The listing builds one solid part. Answer for the finished solid, in the listing's coordinates (mm). A direction names the side the tool comes from. Round coordinates to 2 decimals unless told otherwise and drop trailing zeros. Write each loop counter-clockwise with the first axis right and the second up, starting at its lowest first coordinate (ties: lowest second). Pieces come first, ordered by that corner, then holes.
(1) Each of these flat-tipped pins is pushed along its axis until it touches: pin 1 Ø1.8 at (x, y) = (-24, 10) entering from -Z; pin 2 Ø6.5 at (x, y) = (0, -23.5) entering from +Z; pin 3 Ø1 at (y, z) = (21, 3) entering from +X; pin 4 Ø1.5 at (x, z) = (14.5, 2) entering from +Y. Where does it stop, or does it pass through?
(2) The mould has two halves that part along Y. Classify faces 3 (the face through (26.327, -10.916, 2.465)), 4 (the face through (-26, 0, 2)), 5 (the face through (19, 9, 5)): +Y half, -Y half, draft (parallel to the pull), parting line (faces both ways), or undercut.
(3) Find the intervals of material crossed by probe 1 along Y at (x, z) = (16, 0.65); probe 2 along X at (y, z) = (15.5, 2.85), in increasing order.
(4) A cutting plane is placed at A-A, the plane x = 0. Give the vertices of the cut face in (y, z), and give its area (3 significant figures).
(5) A cutting plane is placed at D-D, the plane z = 1. Give the number of separate pieces and of enclosed holes in the cut face, and give its area (3 significant figures).
(6) For faces 1 (the face through (21, 0, 2)), 2 (the face through (-10.026, -25.564, 0.986)), determine the directions among +Z, -Z, +X, -X, +Y, -Y from which every point of the face is accessible in a straight line to the end or side of a thin tool.
(7) A cutting plane is placed at C-C, the plane x = 11.5. Give the vertices of the cut face in (y, z), and give its area (3 significant figures).
from build123d import *

# Parameters (mm, degrees)
F0_R     = 28.5
F0_R_2   = 2.5
F0_R_3   = 3
F0_R_4   = 20.5
F1_DEPTH = 5
F2_DEPTH = 2


with BuildPart() as f1:
    # F0 (on Top) → F1 (new body)
    with BuildSketch(Plane.XY):
        Circle(F0_R)
        with Locations((-16.6170093579, -16.6170093579)):
            Circle(F0_R_2, mode=Mode.SUBTRACT)
        with Locations((-9.3757440929, -22.6350485465)):
            Circle(F0_R_3, mode=Mode.SUBTRACT)
        with Locations((-22.6350485465, -9.3757440929)):
            Circle(F0_R_3, mode=Mode.SUBTRACT)
        with Locations((0, -23.5)):
            Circle(F0_R_2, mode=Mode.SUBTRACT)
        with Locations((9.3757440929, -22.6350485465)):
            Circle(F0_R_3, mode=Mode.SUBTRACT)
        with Locations((16.6170093579, -16.6170093579)):
            Circle(F0_R_2, mode=Mode.SUBTRACT)
        with Locations((22.6350485465, -9.3757440929)):
            Circle(F0_R_3, mode=Mode.SUBTRACT)
        with Locations((-23.5, 0)):
            Circle(F0_R_2, mode=Mode.SUBTRACT)
        with Locations((-22.6350485465, 9.3757440929)):
            Circle(F0_R_3, mode=Mode.SUBTRACT)
        with Locations((-16.6170093579, 16.6170093579)):
            Circle(F0_R_2, mode=Mode.SUBTRACT)
        with Locations((-9.3757440929, 22.6350485465)):
            Circle(F0_R_3, mode=Mode.SUBTRACT)
        Circle(F0_R_4, mode=Mode.SUBTRACT)
        with Locations((23.5, 0)):
            Circle(F0_R_2, mode=Mode.SUBTRACT)
        with Locations((22.6350485465, 9.3757440929)):
            Circle(F0_R_3, mode=Mode.SUBTRACT)
        with Locations((0, 23.5)):
            Circle(F0_R_2, mode=Mode.SUBTRACT)
        with Locations((9.3757440929, 22.6350485465)):
            Circle(F0_R_3, mode=Mode.SUBTRACT)
        with Locations((16.6170093579, 16.6170093579)):
            Circle(F0_R_2, mode=Mode.SUBTRACT)
        with Locations((-22.6350485465, 9.3757440929)):
            Circle(F0_R_3)
        with Locations((-9.3757440929, 22.6350485465)):
            Circle(F0_R_3)
        with Locations((9.3757440929, 22.6350485465)):
            Circle(F0_R_3)
        with Locations((22.6350485465, 9.3757440929)):
            Circle(F0_R_3)
        with Locations((22.6350485465, -9.3757440929)):
            Circle(F0_R_3)
        with Locations((9.3757440929, -22.6350485465)):
            Circle(F0_R_3)
        with Locations((-9.3757440929, -22.6350485465)):
            Circle(F0_R_3)
        with Locations((-22.6350485465, -9.3757440929)):
            Circle(F0_R_3)
    extrude(amount=F1_DEPTH)

    # F0 (on Top) → F2 (cut)
    with BuildSketch(Plane.XY):
        with Locations((-22.6350485465, -9.3757440929)):
            Circle(F0_R_3)
        with Locations((-9.3757440929, -22.6350485465)):
            Circle(F0_R_3)
        with Locations((9.3757440929, -22.6350485465)):
            Circle(F0_R_3)
        with Locations((22.6350485465, -9.3757440929)):
            Circle(F0_R_3)
        with Locations((22.6350485465, 9.3757440929)):
            Circle(F0_R_3)
        with Locations((9.3757440929, 22.6350485465)):
            Circle(F0_R_3)
        with Locations((-9.3757440929, 22.6350485465)):
            Circle(F0_R_3)
        with Locations((-22.6350485465, 9.3757440929)):
            Circle(F0_R_3)
    extrude(amount=F2_DEPTH, mode=Mode.SUBTRACT)


solid = f1.part
Solutions:
1. pin 1: stops at z = 2
1. pin 2: stops at z = 5
1. pin 3: stops at x = 19.8
1. pin 4: stops at y = 24.96
2. face 3: parting line
2. face 4: undercut
2. face 5: draft
3. probe 1: y = -23.58 to -19.04, -14.19 to -12.82, 12.82 to 14.19, 19.04 to 23.58
3. probe 2: x = -23.92 to -18.85, -14.38 to -13.42, 13.42 to 14.38, 18.85 to 23.92
4. outline: (-28.5, 0) - (-26, 0) - (-26, 5) - (-28.5, 5) - close; (-21, 0) - (-20.5, 0) - (-20.5, 5) - (-21, 5) - close; (20.5, 0) - (21, 0) - (21, 5) - (20.5, 5) - close; (26, 0) - (28.5, 0) - (28.5, 5) - (26, 5) - close
4. area: 30.0 mm2
5. separate pieces: 1
5. enclosed holes: 17
5. area: 848 mm2
6. face 1: +Z, -Z
6. face 2: -Z
7. outline: (-26.08, 0) - (-24.75, 0) - (-24.75, 2) - (-20.52, 2) - (-20.52, 0) - (-16.97, 0) - (-16.97, 5) - (-26.08, 5) - close; (16.97, 0) - (20.52, 0) - (20.52, 2) - (24.75, 2) - (24.75, 0) - (26.08, 0) - (26.08, 5) - (16.97, 5) - close
7. area: 74.1 mm2
